Read the model definition and answer for the solid it produces. Units are mm, in the model's axes. A direction names the side the tool comes from. Coordinates: 2 decimals unless noted, no trailing zeros. Order: outer loops, then holes, each group sorted by start corner. A loop starts at its lowest first (then second) coordinate and runs counter-clockwise, first axis right, second up.
from build123d import *

# Parameters (mm, degrees)
CUT_EXTRUDE1_DEPTH = 1.3
FILLET1_R          = 0.1


with BuildPart() as part:
    # Sketch1 → Revolve1 (revolve)
    with BuildSketch(Plane.XY):
        Polygon((0, 0), (0, 23), (2.75, 23), (2.75, 20), (1.5, 20), (1.5, 0), align=None)
    revolve(axis=Axis((0, 0, 0), (0, 1, 0)))

    # Sketch2 → Cut-Extrude1 (cut)
    with BuildSketch(Plane(origin=(0, 23, 0), x_dir=(1, 0, 0), z_dir=(0, 1, 0))):
        Polygon((0, 1.489563695), (-1.29, 0.744781847), (-1.29, -0.744781847), (0, -1.489563695), (1.29, -0.744781847), (1.29, 0.744781847), align=None)
    extrude(amount=-CUT_EXTRUDE1_DEPTH, mode=Mode.SUBTRACT)

    # Fillet1
    fillet1_edges = [part.edges().sort_by_distance(p)[0] for p in [
        (-2.75, 23, 0),
    ]]
    fillet(fillet1_edges, radius=FILLET1_R)


solid = part.part
Q1. The part is cut by section A-A, the plane z = 0. Determine the outline of the cut face in (x, y), then the cut area to 3 significant figures.
Q2. Which of the six approach directions +Z, -Z, +X, -X, +Y, -Y give full straight-line access (tool end or side, diameter ignored) to faces 1 (the cylindrical face through (-0.596, 21.43, 2.685)), 2 (the flat face through (1.2, 20, 1.2)), 3 (the flat face through (0.64, 22.36, 1.12))?
Q3. Straight lines are drawn through the part: L1, parallel to Y at x = 0.6, z = -1.95; L2, parallel to Y at x = 0.1, z = 0.55; L3, parallel to X at y = 11.5, z = -1.3. For each, find the intervals that lie inside material, in ascending order.
Q4. Determine the mould class of faces 4 (the flat face through (0.654, 22.359, -1.112)), 5 (the cylindrical face through (-1.5, 9.86, -0.07)), 6 (the flat face through (-1.1, 23, 1.1)) for opening direction Z: +Z half, -Z half, draft (parallel to the pull), parting line (faces both ways), or undercut.
Q5. The part is cut by section B-B, the plane y = 20.25. Determine the outline of the cut face in (x, z), then the cut area to 3 significant figures.
Computed values:
1. outline: (-2.75, 20) - (-1.5, 20) - (-1.5, 0) - (1.5, 0) - (1.5, 20) - (2.75, 20) - (2.75, 22.9) arc R0.1 ccw to (2.65, 23) - (1.29, 23) - (1.29, 21.7) - (-1.29, 21.7) - (-1.29, 23) - (-2.65, 23) arc R0.1 ccw to (-2.75, 22.9) - close
1. area: 73.1 mm2
2. face 1: +Y, -Y
2. face 2: -Y
2. face 3: +Y
3. L1: y = 20 to 23
3. L2: y = 0 to 21.7
3. L3: x = -0.75 to 0.75
4. face 4: undercut
4. face 5: parting line
4. face 6: draft
5. outline: circle Ø5.5 at (0, 0)
5. area: 23.8 mm2
